Here's how the part is built. I have some questions about the finished solid (model axes, mm). Coordinates: 2 decimals unless noted, no trailing zeros. Order: outer loops, then holes, each group sorted by start corner. A loop starts at its lowest first (then second) coordinate and runs counter-clockwise, first axis right, second up. Notation, with made-up numbers: M 58,28 L 99,28 A31 cw 99,57 Z; hole C 21.5,0 d6. An arc over 180 degrees is marked long. One line per question, with ' | ' between items. Start each with the question number.
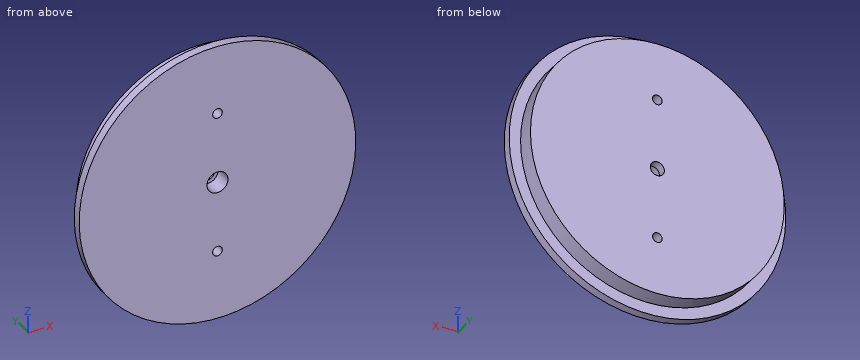
```python
from build123d import *

# Parameters (mm, degrees)
SKETCH1_R           = 79
BOSS_EXTRUDE1_DEPTH = 5
SKETCH2_R           = 72.5
BOSS_EXTRUDE2_DEPTH = 10
SKETCH3_R           = 2.75
CUT_EXTRUDE1_DEPTH  = 113.725329895
SKETCH4_R           = 4
CUT_EXTRUDE2_DEPTH  = 5
SKETCH5_R           = 6
CUT_EXTRUDE3_DEPTH  = 10


with BuildPart() as part:
    # Sketch1 → Boss-Extrude1 (new body)
    with BuildSketch(Plane(origin=(0, 0, 0), x_dir=(1, 0, 0), z_dir=(0, 1, 0))):
        with Locations(Location((0, 0, 0), (0, 0, 270))):
            Circle(SKETCH1_R)
    extrude(amount=BOSS_EXTRUDE1_DEPTH)

    # Sketch2 → Boss-Extrude2 (add)
    with BuildSketch(Plane(origin=(0, 5, 0), x_dir=(1, 0, 0), z_dir=(0, 1, 0))):
        with Locations(Location((0, 0, 0), (0, 0, 270))):
            Circle(SKETCH2_R)
    extrude(amount=BOSS_EXTRUDE2_DEPTH)

    # Sketch3 → Cut-Extrude1 (cut, through all)
    with BuildSketch(Plane(origin=(0, 15, 0), x_dir=(1, 0, 0), z_dir=(0, 1, 0))):
        with Locations(Location((0, 40, 0), (0, 0, 270))):
            Circle(SKETCH3_R)
        with Locations(Location((0, -40, 0), (0, 0, 270))):
            Circle(SKETCH3_R)
    extrude(amount=-CUT_EXTRUDE1_DEPTH, mode=Mode.SUBTRACT)

    # Sketch4 → Cut-Extrude2 (cut)
    with BuildSketch(Plane(origin=(0, 15, 0), x_dir=(1, 0, 0), z_dir=(0, 1, 0))):
        with Locations(Location((0, 0, 0), (0, 0, 270))):
            Circle(SKETCH4_R)
    extrude(amount=-CUT_EXTRUDE2_DEPTH, mode=Mode.SUBTRACT)

    # Sketch5 → Cut-Extrude3 (cut)
    with BuildSketch(Plane.XZ):
        with Locations(Location((0, 0, 0), (0, 0, 270))):
            Circle(SKETCH5_R)
    extrude(amount=-CUT_EXTRUDE3_DEPTH, mode=Mode.SUBTRACT)


solid = part.part
```
1. Imagine slicing it at C-C (y = 8). List the corners of the cut face in (x, z) for me.
2. Imagine slicing it at A-A (x = 0). List the corners of the cut face in (y, z) for me, then the cut area to 4 significant figures.
3. Imagine slicing it at D-D (z = 64.5). List the corners of the cut face in (x, y) for me.
4. Imagine slicing it at B-B (z = 0). List the corners of the cut face in (x, y) for me, then the cut area to 3 significant figures.
5. I need wall thicknesses on line 1 (X direction, y = 3.5, z = 0); line 2 (X direction, y = 5.75, z = -5); line 3 (Y direction, x = -35, z = 64.5). Which ranges of each line are inside material? Lowest first, please.
6. Will these pins go through, and if not, where does the flat tip stop? pin 1 (4 mm diameter, centred on y = 6, z = 53.5, fed in from +X); pin 2 (4 mm diameter, centred on y = 7.5, z = -30, fed in from -X); pin 3 (4 mm diameter, centred on y = 9, z = 4, fed in from -X).
Entries:
1) outline: C 0,0 d145; hole C 0,0 d12; hole C 0,-40 d5.5; hole C 0,40 d5.5
2) outline: M 0,-79 L 5,-79 L 5,-72.5 L 15,-72.5 L 15,-42.75 L 0,-42.75 Z; M 0,-37.25 L 15,-37.25 L 15,-4 L 10,-4 L 10,-6 L 0,-6 Z; M 0,6 L 10,6 L 10,4 L 15,4 L 15,37.25 L 0,37.25 Z; M 0,42.75 L 15,42.75 L 15,72.5 L 5,72.5 L 5,79 L 0,79 Z | area: 1,915 mm²
3) outline: M -45.62,0 L 45.62,0 L 45.62,5 L 33.11,5 L 33.11,15 L -33.11,15 L -33.11,5 L -45.62,5 Z
4) outline: M -79,0 L -6,0 L -6,10 L -4,10 L -4,15 L -72.5,15 L -72.5,5 L -79,5 Z; M 4,10 L 6,10 L 6,0 L 79,0 L 79,5 L 72.5,5 L 72.5,15 L 4,15 Z | area: 2,080 mm²
5) line 1: -79 to -6, 6 to 79 | line 2: -72.33 to -3.32, 3.32 to 72.33 | line 3: 0 to 5
6) pin 1: x = 59.67 | pin 2: x = -66.87 | pin 3: x = -72.47
